Read the model definition and answer for the solid it produces. Units are mm, in the model's axes. A direction names the side the tool comes from. Coordinates: 2 decimals unless noted, no trailing zeros. Order: outer loops, then holes, each group sorted by start corner. A loop starts at its lowest first (then second) coordinate and runs counter-clockwise, first axis right, second up. Notation, with made-up numbers: (9, -13) - (16, -13) arc R5 cw to (16, -5) - close; hole circle Ø9 at (-23.75, -20.75). An arc over 180 degrees is marked (long way). Use one line per item in the form item = value. Start each with the question number.
from build123d import *

# Parameters (mm, degrees)
F0_W     = 76.2
F0_H     = 152.4
F1_DEPTH = 152.4
F2_SIZE  = 147.32
F3_T     = -2.54
F4_R     = 25.4
F5_R     = 5.07999
F6_W     = 15.24
F6_H     = 3.5921024484
F7_DEPTH = 25.4


# Not quite as in the source:
# - a fillet or chamfer is up to 0.001 mm smaller than in the source, because OpenCascade refuses the exact size


with BuildPart() as f1:
    # F0 (on Top) → F1 (new body)
    with BuildSketch(Plane.XY):
        Rectangle(F0_W, F0_H)
    extrude(amount=F1_DEPTH)

    # F2
    f2_edges = [f1.edges().sort_by_distance(p)[0] for p in [
        (0, -76.2, 152.4),
    ]]
    chamfer(f2_edges, length=F2_SIZE)

    # F3
    f3_openings = [f1.faces().sort_by_distance(p)[0] for p in [
        (0, -2.54, 78.74),
    ]]
    offset(amount=F3_T, openings=f3_openings)

    # F4
    f4_edges = [f1.edges().sort_by_distance(p)[0] for p in [
        (0, 73.66, 2.54),
    ]]
    fillet(f4_edges, radius=F4_R)

    # F5 (radius 5.08 in the source; OpenCascade refuses exactly that, so slightly less here)
    f5_edges = [f1.edges().sort_by_distance(p)[0] for p in [
        (0, -73.66, 2.54),
    ]]
    fillet(f5_edges, radius=F5_R)

    # F6 (on face) → F7 (join)
    with BuildSketch(Plane(origin=(0, -40.64, 40.64), x_dir=(1, 0, 0), z_dir=(0, -0.7071067812, 0.7071067812))):
        with Locations((-27.94, -48.4933830538)):
            Rectangle(F6_W, F6_H)
        with Locations((27.94, -48.4933830538)):
            Rectangle(F6_W, F6_H)
        with Locations((0.0408754674, -48.4933830538)):
            Rectangle(F6_W, F6_H)
    extrude(amount=F7_DEPTH)


solid = f1.part
Q1. A cutting plane is placed at D-D (z = 31). Give the vertices of the cut face in (x, y).
Q2. A cutting plane is placed at A-A (y = -83.5). Give the vertices of the cut face in (x, z).
Q3. Given P1, Ø10, axis at x = 24, y = -3.5, coming from the +Z side; P2, Ø2.5, axis at x = -6, z = 2, coming from the -Y side; P3, Ø22.5, axis at y = -82, z = 20.5, coming from the +X side, each flat-ended and moving along its own axis, determine where each tip first touches the part or whether it passes through.
Q4. A cutting plane is placed at C-C (y = 0.5). Give the vertices of the cut face in (x, z).
Q5. For a pull along Z with two mould halves and no side action, classify faces 4 (the flat face through (-1, 1, 0)), 5 (the flat face through (0, 71, 149.86)), 6 (the flat face through (38.1, 16, 58)) as +Z half, -Z half, draft (parallel to the pull), parting line (faces both ways), or undercut.
Q6. Which of the six approach directions +Z, -Z, +X, -X, +Y, -Y give full straight-line access (tool end or side, diameter ignored) to faces 1 (the cylindrical face through (0.498, -72.132, 3.989)), 2 (the flat face through (27.83, -82.51, 16.47)), 3 (the flat face through (-1, -76.2, 3))?
Q7. Consider probe 1 along X at (y, z) = (41.5, 57.5); probe 2 along Y at (x, z) = (-22.5, 130.5); probe 3 along Z at (x, y) = (34.5, 19). Determine where each line is inside the solid, lowest interval first.
Q8. A cutting plane is placed at B-B (z = 12.5). Give the vertices of the cut face in (x, y), then the cut area to 3 significant figures.
Result sheet:
q1.outline = (-38.1, -50.28) - (-35.56, -50.28) - (-35.56, 73.66) - (35.56, 73.66) - (35.56, -50.28) - (38.1, -50.28) - (38.1, 76.2) - (-38.1, 76.2) - close
q2.outline = (-35.56, 12.38) - (-20.32, 12.38) - (-20.32, 17.46) - (-35.56, 17.46) - close; (-7.58, 12.38) - (7.66, 12.38) - (7.66, 17.46) - (-7.58, 17.46) - close; (20.32, 12.38) - (35.56, 12.38) - (35.56, 17.46) - (20.32, 17.46) - close
q3.P1 = 2.54
q3.P2 = -76.2
q3.P3 = 35.56
q4.outline = (-38.1, 0) - (38.1, 0) - (38.1, 81.78) - (35.56, 81.78) - (35.56, 2.54) - (-35.56, 2.54) - (-35.56, 81.78) - (-38.1, 81.78) - close
q5.face_4 = -Z half
q5.face_5 = undercut
q5.face_6 = draft
q6.face_1 = +Z
q6.face_2 = +Z, +X, -X
q6.face_3 = -Z, +X, -X, -Y
q7.probe_1 = -38.1 to -35.56, 35.56 to 38.1
q7.probe_2 = 73.66 to 76.2
q7.probe_3 = 0 to 2.54
q8.outline = (-38.1, -68.78) - (-35.56, -68.78) - (-35.56, 68.43) - (35.56, 68.43) - (35.56, -68.78) - (38.1, -68.78) - (38.1, 76.2) - (-38.1, 76.2) - close; (-35.56, -83.62) - (-20.32, -83.62) - (-20.32, -78.54) - (-35.56, -78.54) - close; (-7.58, -83.62) - (7.66, -83.62) - (7.66, -78.54) - (-7.58, -78.54) - close; (20.32, -83.62) - (35.56, -83.62) - (35.56, -78.54) - (20.32, -78.54) - close
q8.area = 1,520 mm^2
